Could you check a few things on this model? Use its own coordinates, in mm. Face numbers are marked on the shaded views. Round coordinates to 2 decimals unless told otherwise and drop trailing zeros. Write each loop counter-clockwise with the first axis right and the second up, starting at its lowest first coordinate (ties: lowest second). Pieces come first, ordered by that corner, then holes. Notation, with made-up numbers: (-26, 29) -> (12, 29) arc R16 ccw to (12, 51) -> close; hole circle Ø6 at (-2.5, 66.5). An arc over 180 degrees is marked (long way). One line per question, with ' | ' between items. Start each with the question number.
1. Thinking about a two-plate mould opening in X: for the marked faces 1, 2, 3 and 4, which applies, released by +X, released by -X, zero draft, split by the parting line, or undercut?
2. Imagine slicing it at D-D, the plane z = 5. List the corners of the cut face in (x, y) for me (1 decimal).
3. Imagine slicing it at C-C, the plane z = 9. List the corners of the cut face in (x, y) for me (1 decimal).
4. Imagine slicing it at A-A, the plane x = 0. List the corners of the cut face in (y, z) for me (3 decimals).
5. If I drill on line 1 along Y through (x, z) = (0, -10) (3 decimals); line 2 along Z through (x, y) = (0, -21.75) (3 decimals); line 3 along Y through (x, z) = (0.5, 4) (3 decimals), over which ranges is the centre line in solid material (lowest first)? Write a range as [from, to].
6. For pin 1 Ø1.6 at (x, z) = (5.66, 5.66) entering from -Y (3 decimals); pin 2 Ø4 at (x, y) = (0, 0.635) entering from -Z, each with a flat end and sliding along its axis, tell me the tip position at first contact or that it passes through.
7. Imagine slicing it at B-B, the plane y = -13. List the corners of the cut face in (x, z) for me (3 decimals), and give its area (3 significant figures).
from build123d import *

# Parameters (mm, degrees)
SKETCH1_W               = 25.4
SKETCH1_H               = 25.4
BOSS_EXTRUDE1_DEPTH     = 28.575
SKETCH2_R               = 3.175
CUT_EXTRUDE1_DEPTH      = 16.51
SKETCH5_R               = 2.38125
CUT_EXTRUDE3_DEPTH      = 13.7
CUT_EXTRUDE3_DEPTH_BACK = 13.7
CHAMFER1_SIZE           = 0.79375
SKETCH6_R               = 1.35255
CUT_EXTRUDE4_DEPTH      = 6.35


with BuildPart() as part:
    # Sketch1 → Boss-Extrude1 (new body, symmetric)
    with BuildSketch(Plane(origin=(0, 0, 0), x_dir=(1, 0, 0), z_dir=(0, 1, 0))):
        Rectangle(SKETCH1_W, SKETCH1_H)
    extrude(amount=BOSS_EXTRUDE1_DEPTH, both=True)

    # Sketch2 → Cut-Extrude1 (cut)
    with BuildSketch(Plane(origin=(0, -28.575, 0), x_dir=(-1, 0, 0), z_dir=(0, -1, 0))):
        Circle(SKETCH2_R)
    extrude(amount=-CUT_EXTRUDE1_DEPTH, mode=Mode.SUBTRACT)

    # Sketch5 → Cut-Extrude3 (cut, two sides)
    with BuildSketch(Plane.XY) as cut_extrude3_sk:
        with Locations((0, 0.635)):
            Circle(SKETCH5_R)
        with Locations((0, 19.685)):
            Circle(SKETCH5_R)
    extrude(amount=CUT_EXTRUDE3_DEPTH, mode=Mode.SUBTRACT)
    extrude(cut_extrude3_sk.sketch, amount=-CUT_EXTRUDE3_DEPTH_BACK, mode=Mode.SUBTRACT)

    # Chamfer1
    chamfer1_edges = [part.edges().sort_by_distance(p)[0] for p in [
        (-12.7, 28.575, 0),
        (0, 28.575, 12.7),
        (12.7, 28.575, 0),
        (0, -28.575, 12.7),
        (-12.7, -28.575, 0),
        (0, -28.575, -12.7),
        (12.7, -28.575, 0),
        (0, 28.575, -12.7),
    ]]
    chamfer(chamfer1_edges, length=CHAMFER1_SIZE)

    # Sketch6 → Cut-Extrude4 (cut)
    with BuildSketch(Plane(origin=(0, -28.575, 0), x_dir=(-1, 0, 0), z_dir=(0, -1, 0))):
        with Locations((-5.656854249, 5.656854249)):
            Circle(SKETCH6_R)
        with Locations((5.656854249, 5.656854249)):
            Circle(SKETCH6_R)
        with Locations((5.656854249, -5.656854249)):
            Circle(SKETCH6_R)
        with Locations((-5.656854249, -5.656854249)):
            Circle(SKETCH6_R)
    extrude(amount=-CUT_EXTRUDE4_DEPTH, mode=Mode.SUBTRACT)


solid = part.part
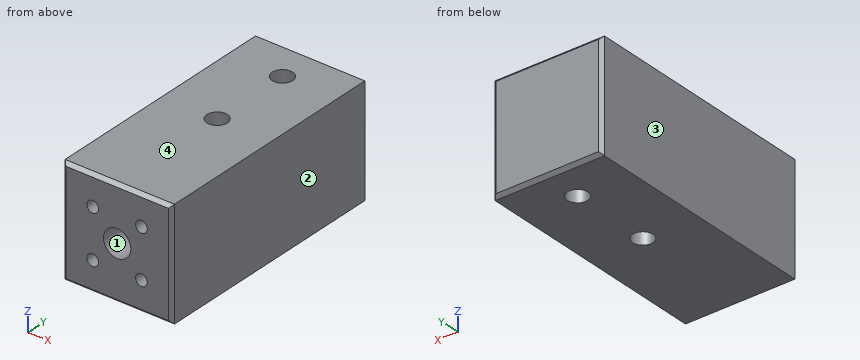
Geometry results:
1) face 1: undercut | face 2: released by +X | face 3: released by -X | face 4: zero draft
2) outline: (-12.7, -27.8) -> (-11.9, -28.6) -> (-6.8, -28.6) -> (-6.8, -22.2) -> (-4.5, -22.2) -> (-4.5, -28.6) -> (4.5, -28.6) -> (4.5, -22.2) -> (6.8, -22.2) -> (6.8, -28.6) -> (11.9, -28.6) -> (12.7, -27.8) -> (12.7, 27.8) -> (11.9, 28.6) -> (-11.9, 28.6) -> (-12.7, 27.8) -> close; hole circle Ø4.8 at (0, 0.6); hole circle Ø4.8 at (0, 19.7)
3) outline: (-12.7, -27.8) -> (-11.9, -28.6) -> (11.9, -28.6) -> (12.7, -27.8) -> (12.7, 27.8) -> (11.9, 28.6) -> (-11.9, 28.6) -> (-12.7, 27.8) -> close; hole circle Ø4.8 at (0, 0.6); hole circle Ø4.8 at (0, 19.7)
4) outline: (-28.575, -11.906) -> (-27.781, -12.7) -> (-1.746, -12.7) -> (-1.746, 12.7) -> (-27.781, 12.7) -> (-28.575, 11.906) -> (-28.575, 3.175) -> (-12.065, 3.175) -> (-12.065, -3.175) -> (-28.575, -3.175) -> close; (3.016, -12.7) -> (17.304, -12.7) -> (17.304, 12.7) -> (3.016, 12.7) -> close; (22.066, -12.7) -> (27.781, -12.7) -> (28.575, -11.906) -> (28.575, 11.906) -> (27.781, 12.7) -> (22.066, 12.7) -> close
5) line 1: y = [-28.575, -1.746], [3.016, 17.304], [22.066, 28.575] | line 2: z = [-12.7, -3.175], [3.175, 12.7] | line 3: y = [-28.575, -1.693], [2.963, 17.357], [22.013, 28.575]
6) pin 1: stops at y = -22.225 | pin 2: passes through
7) outline: (-12.7, -12.7) -> (12.7, -12.7) -> (12.7, 12.7) -> (-12.7, 12.7) -> close; hole circle Ø6.35 at (0, 0) | area: 613 mm2
